```python
from build123d import *

# Parameters (mm, degrees)
CHAMFER1_SIZE      = 0.5
SKETCH2_R          = 3
CUT_EXTRUDE1_DEPTH = 20.595917942
SKETCH3_R          = 1.5
CUT_EXTRUDE2_DEPTH = 20.595917942
SKETCH4_R          = 1.5
CUT_EXTRUDE3_DEPTH = 20.595918106
FILLET1_R          = 0.2


with BuildPart() as part:
    # Sketch1 → Revolve1 (revolve)
    with BuildSketch(Plane.XY, mode=Mode.PRIVATE) as revolve1_sk:
        Polygon((0, 0), (8, 0), (8, 1), (6, 1), (6, 8), (8, 8), (8, 16), (0, 16), align=None)
    revolve(revolve1_sk.sketch.rotate(Axis((0, 16, 0), (0, -1, 0)), 180), axis=Axis((0, 16, 0), (0, -1, 0)))

    # Chamfer1
    chamfer1_edges = [part.edges().sort_by_distance(p)[0] for p in [
        (8, 1, 0),
    ]]
    chamfer(chamfer1_edges, length=CHAMFER1_SIZE)

    # Sketch2 → Cut-Extrude1 (cut, through all)
    with BuildSketch(Plane(origin=(0, 16, 0), x_dir=(1, 0, 0), z_dir=(0, 1, 0))):
        with Locations(Location((0, 0, 0), (0, 0, 180))):
            Circle(SKETCH2_R)
    extrude(amount=-CUT_EXTRUDE1_DEPTH, mode=Mode.SUBTRACT)

    # Sketch3 → Cut-Extrude2 (cut, through all)
    with BuildSketch(Plane(origin=(0, 0, 0), x_dir=(0, 0, -1), z_dir=(1, 0, 0))):
        with Locations(Location((0, 12, 0), (0, 0, 89.999999999))):
            Circle(SKETCH3_R)
    extrude(amount=-CUT_EXTRUDE2_DEPTH, mode=Mode.SUBTRACT)

    # Sketch4 → Cut-Extrude3 (cut, through all)
    with BuildSketch(Plane.XY):
        with Locations((0, 12)):
            Circle(SKETCH4_R)
    extrude(amount=-CUT_EXTRUDE3_DEPTH, mode=Mode.SUBTRACT)

    # Fillet1
    fillet1_edges = [part.edges().sort_by_distance(p)[0] for p in [
        (8, 16, 0),
        (8, 8, 0),
    ]]
    fillet(fillet1_edges, radius=FILLET1_R)


solid = part.part
```
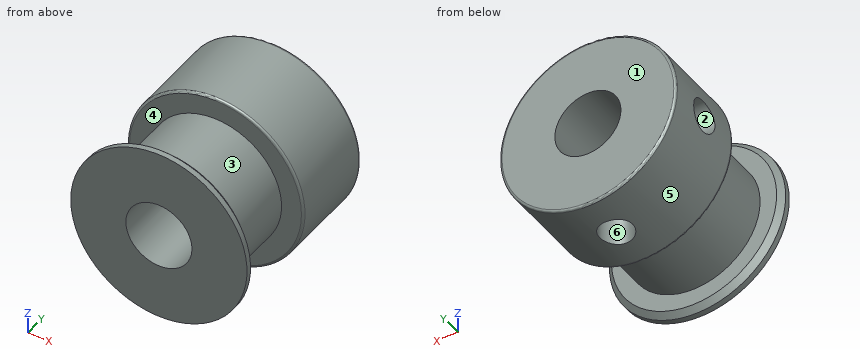
Work out the finished part from the listing and answer in its coordinate system (mm). Face numbers are marked on the shaded views. A direction names the side the tool comes from. Round coordinates to 2 decimals unless told otherwise and drop trailing zeros. Write each loop counter-clockwise with the first axis right and the second up, starting at its lowest first coordinate (ties: lowest second). Pieces come first, ordered by that corner, then holes. Notation, with made-up numbers: (40.25, 17.25) - (85.25, 17.25) arc R20 ccw to (85.25, 55.25) - close; hole circle Ø7 at (69.25, -15). An arc over 180 degrees is marked (long way). Return JSON: item names as keys, results as strings. Group by question number.
Q1. For the marked faces 1, 2 and 3, determine the directions among +Z, -Z, +X, -X, +Y, -Y from which every point of the face is accessible in a straight line to the end or side of a thin tool.
Q2. The mould has two halves that part along X. Classify the marked faces 4, 5 and 6: released by +X, released by -X, zero draft, split by the parting line, or undercut.
Q3. Each of these flat-tipped pins is pushed along its axis until it touches: pin 1 Ø6 at (x, y) = (3.5, 13.5) entering from -Z; pin 2 Ø1.8 at (y, z) = (12, 0) entering from -X; pin 3 Ø1.5 at (y, z) = (2, 3.5) entering from -X. Where does it stop, or does it pass through?
Q4. The part is cut by section C-C on y = 12. Write down the section's boundary in (x, z).
Q5. The part is cut by section B-B on x = 0. Write down the section's boundary in (y, z), then the cut area to 3 significant figures.
Q6. Find the intervals of material crossed by L1, parallel to Y at x = -2.5, z = -6; L2, parallel to Z at x = 0, y = 9.75; L3, parallel to Y at x = -6, z = 0.75, in increasing order.
Q7. The part is cut by section A-A on z = 0. Write down the section's boundary in (x, y), then the cut area to 3 significant figures.
Q8. The part is cut by section D-D on y = 8.5. Write down the section's boundary in (x, z).
Solved:
{
 "1": {"face 1": "+Z, -Z, +X, -X, +Y", "face 2": "-X", "face 3": "none"},
 "2": {"face 4": "zero draft", "face 5": "split by the parting line", "face 6": "undercut"},
 "3": {"pin 1": "z = -7.98", "pin 2": "x = 2.86", "pin 3": "x = -5.33"},
 "4": {"outline": "(-7.86, -1.5) arc R8 ccw to (-1.5, -7.86) - (-1.5, -2.6) arc R3 cw to (-2.6, -1.5) - close; (-7.86, 1.5) - (-2.6, 1.5) arc R3 cw (long way) to (1.5, -2.6) - (1.5, -7.86) arc R8 ccw (long way) to start"},
 "5": {"outline": "(0, -8) - (0.5, -8) - (1, -7.5) - (1, -6) - (8, -6) - (8, -7.8) arc R0.2 ccw to (8.2, -8) - (10.5, -8) - (10.5, -3) - (0, -3) - close; (0, 3) - (16, 3) - (16, 7.8) arc R0.2 ccw to (15.8, 8) - (8.2, 8) arc R0.2 ccw to (8, 7.8) - (8, 6) - (1, 6) - (1, 7.5) - (0.5, 8) - (0, 8) - close; (13.5, -8) - (15.8, -8) arc R0.2 ccw to (16, -7.8) - (16, -3) - (13.5, -3) - close", "area": "117 mm²"},
 "6": {"L1": "0 to 1, 8 to 16", "L2": "-8 to -3, 3 to 8", "L3": "0 to 1, 8 to 10.7, 13.3 to 16"},
 "7": {"outline": "(-8, 0) - (-3, 0) - (-3, 10.5) - (-8, 10.5) - (-8, 8.2) arc R0.2 ccw to (-7.8, 8) - (-6, 8) - (-6, 1) - (-7.5, 1) - (-8, 0.5) - close; (-8, 13.5) - (-3, 13.5) - (-3, 16) - (-7.8, 16) arc R0.2 ccw to (-8, 15.8) - close; (3, 0) - (8, 0) - (8, 0.5) - (7.5, 1) - (6, 1) - (6, 8) - (7.8, 8) arc R0.2 ccw to (8, 8.2) - (8, 15.8) arc R0.2 ccw to (7.8, 16) - (3, 16) - close", "area": "117 mm²"},
 "8": {"outline": "circle Ø16 at (0, 0); hole circle Ø6 at (0, 0)"}
}
